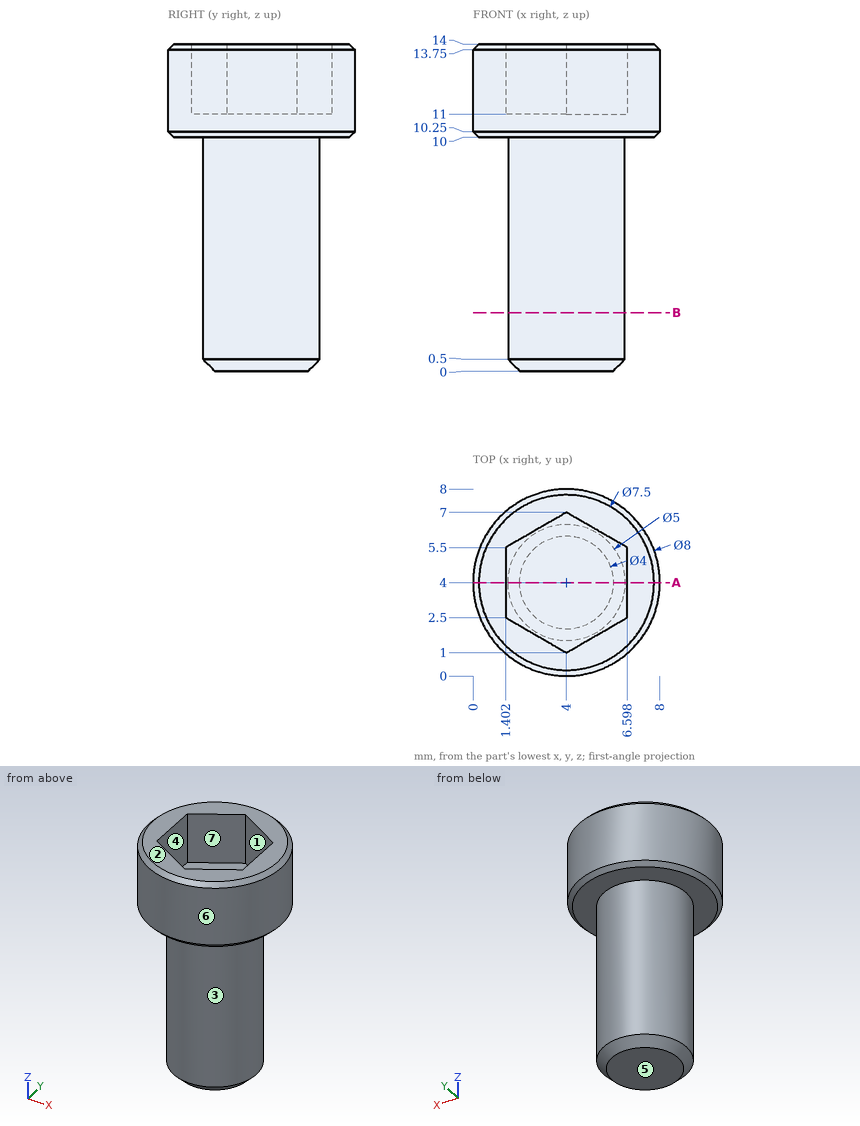
Job drawing, mm, ordinate dimensions from the low corner. One solid piece. A direction names the side the tool comes from. Coordinates: 2 decimals unless noted, no trailing zeros. Order: outer loops, then holes, each group sorted by start corner. A loop starts at its lowest first (then second) coordinate and runs counter-clockwise, first axis right, second up. Notation, with made-up numbers: M -15.5,79 L 25.5,79 A19 ccw 25.5,116 Z; hole C -10.5,79.25 d6. An arc over 180 degrees is marked long. One line per question, with ' | ' between items.
Q1. 3-axis set-ups, long thin cutter, end or side, ignore diameter. For the marked faces 1, 2 and 3: which of +Z, -Z, +X, -X, +Y, -Y reach the whole face in a straight line?
A:
face 1: +Z | face 2: +Z, +X, -X, +Y, -Y | face 3: -Z
Q2. Slice it at A-A (y = 4). Give the cut face in (x, z).
A:
outline: M 0,10.25 L 0.25,10 L 1.5,10 L 1.5,0.5 L 2,0 L 6,0 L 6.5,0.5 L 6.5,10 L 7.75,10 L 8,10.25 L 8,13.75 L 7.75,14 L 6.6,14 L 6.6,11 L 1.4,11 L 1.4,14 L 0.25,14 L 0,13.75 Z
Q3. Pin check, flat tips, straight feed: P1, Ø2.5, axis at x = 4.5, y = 3.5, coming from the +Z side; P2, Ø4, axis at x = 6.5, z = 8.5, coming from the -Y side (3 decimals). Stop position of each tip, or through.
A:
P1: stops at z = 11 | P2: stops at y = 0.305
Q4. Drill centre lines: line 1 (X direction, y = 6, z = 4.5); line 2 (Z direction, x = 1.25, y = 3.5); line 3 (X direction, y = 3.5, z = 13). Where is each one in solid material? Low to high.
A:
line 1: x = 2.5 to 5.5 | line 2: z = 10 to 14 | line 3: x = 0.03 to 1.4, 6.6 to 7.97
Q5. Two-plate mould, pull along X, no slides. Class the marked faces 4, 5, 6 and 7: +X half, -X half, draft (parallel to the pull), parting line (faces both ways), or undercut.
A:
face 4: undercut | face 5: draft | face 6: parting line | face 7: undercut
Q6. Slice it at B-B (z = 2.5). Give the cut face in (x, y), and give its area (3 significant figures).
A:
outline: C 4,4 d5 | area: 19.6 mm^2
